Input: part model. Units: mm. Frame: model coordinates. Face numbers are marked on the shaded views. Coordinates: 2 decimals unless noted, no trailing zeros. Write each loop counter-clockwise with the first axis right and the second up, starting at its lowest first coordinate (ties: lowest second). Pieces come first, ordered by that corner, then holes. Notation, with made-up numbers: (-39.5, 17) - (-20.5, 17) arc R12 cw to (-20.5, 22) - close; hole circle Ø3 at (26.5, 38.5). An arc over 180 degrees is marked (long way). Put each result on its own line as item: value. Start each with the question number.
1. Cut plane B-B, the plane x = -2. Return loops of the section in (y, z).
2. Cut plane A-A, the plane z = 0. Return loops of the section in (x, y) (3 decimals).
3. Pull-direction query (Z, two-part tool) for the marked faces 1 and 2; classes: released by +Z, released by -Z, zero draft, split by the parting line, or undercut.
4. Pin query (flat end, axial travel): pin 1 (4 mm diameter, centred on x = 2, y = 62, fed in from -Z); pin 2 (1.5 mm diameter, centred on y = 69, z = -35, fed in from -X); pin 3 (5 mm diameter, centred on x = 6, z = -42, fed in from +Y). Return the tip coordinate at first contact, or that it passes through.
5. Line query: line 1 (Z direction, x = 6.25, y = 32); line 2 (Z direction, x = 0.75, y = 38); line 3 (X direction, y = 41, z = -5.5). Output: solid intervals per line, ascending.
6. Cut plane D-D, the plane z = -19. Return loops of the section in (x, y).
7. Cut plane C-C, the plane x = 8.5. Count the separate pieces of the cut face and the enclosed holes in it, and give its area (3 significant figures).
from build123d import *

# Parameters (mm, degrees)
SKETCH1_R                   = 89.825
SKETCH1_R_2                 = 47.825
BOSS_EXTRUDE1_DEPTH         = 10
SKETCH3_R                   = 47.825
TBH_IDK_DEPTH               = 5
EXTRUSION_START             = 5
SKETCH4_R                   = 47.825
EXTRUSION_TO_FUEL_MAN_DEPTH = 5
OX_DOWNCOMER_REACH          = 129.914
OX_PROFILE_R                = 1.5
OX_ORIFICES_COUNT           = 3
SKETCH7_R                   = 47.825
FUEL_BLOCKERS_DEPTH         = 5
SKETCH8_R                   = 25.085
TI_CUT_EXTRUDE_DEPTH        = 128.424727781
SKETCH9_R                   = 51.325
FUEL_VOLUME_DEPTH           = 2
SKETCH10_R                  = 5
CUT_EXTRUDE1_DEPTH          = 128.91427305
SKETCH12_W                  = 10
SKETCH12_H                  = 179.65
CUT_EXTRUDE2_DEPTH          = 150.516390415


with BuildPart() as part:
    # Sketch1 → Boss-Extrude1 (new body)
    with BuildSketch(Plane(origin=(0, 0, 0), x_dir=(0, 0, -1), z_dir=(1, 0, 0))):
        Circle(SKETCH1_R)
        Circle(SKETCH1_R_2, mode=Mode.SUBTRACT)
    extrude(amount=BOSS_EXTRUDE1_DEPTH)

    # Sketch3 → tbh idk (add)
    with BuildSketch(Plane.ZY):
        Circle(SKETCH3_R)
    extrude(amount=-TBH_IDK_DEPTH)

    # Sketch4 → Extrusion to Fuel Man (add)
    with BuildSketch(Plane.ZY.offset(EXTRUSION_START)):
        Circle(SKETCH4_R)
    extrude(amount=-EXTRUSION_TO_FUEL_MAN_DEPTH)

    # Ox Profile → Ox Downcomer (cut, up to next)
    with BuildSketch(Plane.ZY.offset(5), mode=Mode.PRIVATE) as ox_downcomer_sk1:
        with Locations((11.464101615, 29.2826)):
            Circle(OX_PROFILE_R)
    ox_downcomer_tool1 = extrude(ox_downcomer_sk1.sketch, amount=-OX_DOWNCOMER_REACH, mode=Mode.PRIVATE) & part.part
    # Ox Profile → Ox Downcomer (cut, up to next)
    with BuildSketch(Plane.ZY.offset(5), mode=Mode.PRIVATE) as ox_downcomer_sk2:
        with Locations((-11.464101615, 29.2826)):
            Circle(OX_PROFILE_R)
    ox_downcomer_tool2 = extrude(ox_downcomer_sk2.sketch, amount=-OX_DOWNCOMER_REACH, mode=Mode.PRIVATE) & part.part
    ox_downcomer_1 = ox_downcomer_tool1.solids().sort_by_distance((-5, 29.2826, 11.464102))[0]
    add(ox_downcomer_1, mode=Mode.SUBTRACT)
    ox_downcomer_2 = ox_downcomer_tool2.solids().sort_by_distance((-5, 29.2826, -11.464102))[0]
    add(ox_downcomer_2, mode=Mode.SUBTRACT)
    ox_downcomer = ox_downcomer_1 + ox_downcomer_2  # Ox Downcomer as one shape, for the pattern or mirror that repeats it

    # Ox Orifices: Ox Downcomer ×3 about axis
    ox_orifices_axis = Axis((0, -0.057725471, 0), (1, 0, 0))
    for i in range(1, OX_ORIFICES_COUNT):
        add(ox_downcomer.rotate(ox_orifices_axis, i * 360 / OX_ORIFICES_COUNT), mode=Mode.SUBTRACT)

    # Sketch7 → Fuel Blockers (cut)
    with BuildSketch(Plane.ZY.offset(5)):
        Circle(SKETCH7_R)
        with BuildLine():
            Line((-34.988640613, -2.46309677), (-15.361215932, 31.5326))
            ThreePointArc((-15.361215932, 31.5326), (-10.299415912, 33.629266218), (-6.964101615, 29.2826))
            ThreePointArc((-6.964101615, 29.2826), (0, 22.318498385), (6.964101615, 29.2826))
            ThreePointArc((6.964101615, 29.2826), (10.299415912, 33.629266218), (15.361215932, 31.5326))
            Line((15.361215932, 31.5326), (34.988640613, -2.46309677))
            ThreePointArc((34.988640613, -2.46309677), (34.273506812, -7.895077285), (28.841526296, -8.610211087))
            ThreePointArc((28.841526296, -8.610211087), (19.328386576, -11.159249192), (21.877424681, -20.672388913))
            ThreePointArc((21.877424681, -20.672388913), (23.9740909, -25.734188933), (19.627424681, -29.06950323))
            Line((19.627424681, -29.06950323), (-19.627424681, -29.06950323))
            ThreePointArc((-19.627424681, -29.06950323), (-23.9740909, -25.734188933), (-21.877424681, -20.672388913))
            ThreePointArc((-21.877424681, -20.672388913), (-19.328386576, -11.159249192), (-28.841526296, -8.610211087))
            ThreePointArc((-28.841526296, -8.610211087), (-34.273506812, -7.895077285), (-34.988640613, -2.46309677))
        make_face(mode=Mode.SUBTRACT)
    extrude(amount=-FUEL_BLOCKERS_DEPTH, mode=Mode.SUBTRACT)

    # Sketch8 → TI Cut Extrude (cut, through all)
    with BuildSketch(Plane(origin=(5, 0, 0), x_dir=(0, 0, -1), z_dir=(1, 0, 0))):
        Circle(SKETCH8_R)
    extrude(amount=-TI_CUT_EXTRUDE_DEPTH, mode=Mode.SUBTRACT)

    # Sketch9 → Fuel Volume (cut)
    with BuildSketch(Plane.ZY):
        Circle(SKETCH9_R)
        with BuildLine():
            ThreePointArc((-15.361215932, 31.5326), (-10.299415912, 33.629266218), (-6.964101615, 29.2826))
            ThreePointArc((-6.964101615, 29.2826), (-6.485666055, 26.745899952), (-5.116096664, 24.557743787))
            ThreePointArc((-5.116096664, 24.557743787), (0, 25.085), (5.116096664, 24.557743787))
            ThreePointArc((5.116096664, 24.557743787), (6.485666055, 26.745899952), (6.964101615, 29.2826))
            ThreePointArc((6.964101615, 29.2826), (10.299415912, 33.629266218), (15.361215932, 31.5326))
            Line((15.361215932, 31.5326), (34.988640613, -2.46309677))
            ThreePointArc((34.988640613, -2.46309677), (34.273506812, -7.895077285), (28.841526296, -8.610211087))
            ThreePointArc((28.841526296, -8.610211087), (26.405461833, -7.756198412), (23.825678311, -7.848202214))
            ThreePointArc((23.825678311, -7.848202214), (21.724247254, -12.5425), (18.709581647, -16.709541573))
            ThreePointArc((18.709581647, -16.709541573), (19.919795778, -18.98970154), (21.877424681, -20.672388913))
            ThreePointArc((21.877424681, -20.672388913), (23.9740909, -25.734188933), (19.627424681, -29.06950323))
            Line((19.627424681, -29.06950323), (-19.627424681, -29.06950323))
            ThreePointArc((-19.627424681, -29.06950323), (-23.9740909, -25.734188933), (-21.877424681, -20.672388913))
            ThreePointArc((-21.877424681, -20.672388913), (-19.919795778, -18.98970154), (-18.709581647, -16.709541573))
            ThreePointArc((-18.709581647, -16.709541573), (-21.724247254, -12.5425), (-23.825678311, -7.848202214))
            ThreePointArc((-23.825678311, -7.848202214), (-26.405461833, -7.756198412), (-28.841526296, -8.610211087))
            ThreePointArc((-28.841526296, -8.610211087), (-34.273506812, -7.895077285), (-34.988640613, -2.46309677))
            Line((-34.988640613, -2.46309677), (-15.361215932, 31.5326))
        make_face(mode=Mode.SUBTRACT)
    extrude(amount=-FUEL_VOLUME_DEPTH, mode=Mode.SUBTRACT)

    # Sketch10 → Cut-Extrude1 (cut, through all)
    with BuildSketch(Plane(origin=(10, 0, 0), x_dir=(0, 0, -1), z_dir=(1, 0, 0))):
        with Locations((0, 68.825)):
            Circle(SKETCH10_R)
        with Locations((59.604198415, 34.4125)):
            Circle(SKETCH10_R)
        with Locations((59.604198415, -34.4125)):
            Circle(SKETCH10_R)
        with Locations((0, -68.825)):
            Circle(SKETCH10_R)
        with Locations((-59.604198415, -34.4125)):
            Circle(SKETCH10_R)
        with Locations((-59.604198415, 34.4125)):
            Circle(SKETCH10_R)
    extrude(amount=-CUT_EXTRUDE1_DEPTH, mode=Mode.SUBTRACT)

    # Sketch12 → Cut-Extrude2 (cut, through all)
    with BuildSketch(Plane(origin=(0, 29.2826, 0), x_dir=(1, 0, 0), z_dir=(0, 1, 0))):
        with Locations((5, 0)):
            Rectangle(SKETCH12_W, SKETCH12_H)
        Polygon((-5, -34.988640613), (-5, -35.591526296), (0, -35.591526296), (0, 35.591526296), (-5, 35.591526296), (-5, 34.988640613), (-5, 28.841526296), (-5, 18.709581647), (-5, 15.361215932), (-5, -6.964101615), (-5, -15.361215932), (-5, -18.709581647), (-5, -28.841526296), align=None)
    extrude(amount=-CUT_EXTRUDE2_DEPTH, mode=Mode.SUBTRACT)


solid = part.part
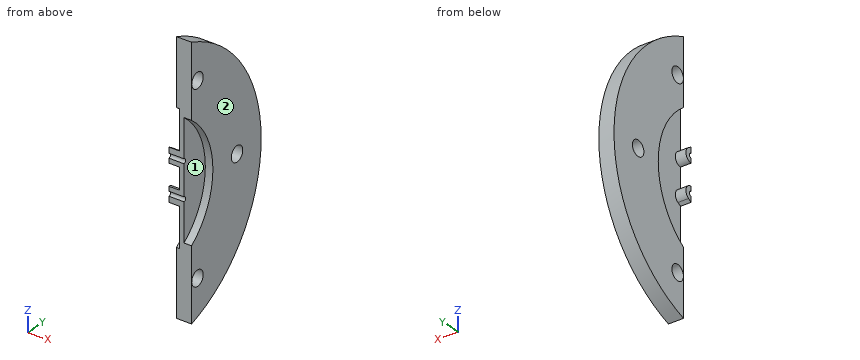
Report:
1. outline: (29.28, -16.66) - (31.53, -15.36) arc R4.5 ccw to (29.28, -6.96) - (29.28, -9.96) arc R1.5 cw to (29.28, -12.96) - close; (29.28, 6.96) arc R4.5 ccw to (31.53, 15.36) - (29.28, 16.66) - (29.28, 12.96) arc R1.5 cw to (29.28, 9.96) - close
2. outline: (0, 51.325) - (2, 51.325) - (2, 29.283) - (5, 29.283) - (5, 47.825) - (10, 47.825) - (10, 63.825) - (0, 63.825) - close; (0, 73.825) - (10, 73.825) - (10, 89.825) - (0, 89.825) - close
3. face 1: undercut
3. face 2: zero draft
4. pin 1: stops at z = -66.85
4. pin 2: stops at x = 0
4. pin 3: stops at y = 80.67
5. line 1: z = -83.93 to -63.98, -55.22 to -35.54, 35.54 to 55.22, 63.98 to 83.93
5. line 2: z = -81.39 to -63.09, -56.12 to -34.5, 34.5 to 56.12, 63.09 to 81.39
5. line 3: x = 2 to 5
6. outline: (0, 47.68) - (2, 47.68) - (2, 29.28) - (5, 29.28) - (5, 43.89) - (10, 43.89) - (10, 87.79) - (0, 87.79) - close
7. separate pieces: 1
7. enclosed holes: 3
7. area: 6,290 mm^2
